Here's how the part is built. I have some questions about the finished solid (model axes, mm). Face numbers are marked on the shaded views. A direction names the side the tool comes from. Round coordinates to 2 decimals unless told otherwise and drop trailing zeros. Order: outer loops, then holes, each group sorted by start corner. A loop starts at its lowest first (then second) coordinate and runs counter-clockwise, first axis right, second up. Notation, with made-up numbers: (43, 80) -> (101, 80) arc R19 cw to (101, 111) -> close; hole circle Ø4 at (42.5, -0.5). An arc over 180 degrees is marked (long way). Use a Markdown table: item, result. Add a question column.
(1) I want a section at A-A, the plane y = 35.5. Please give me the cut outline in (x, z).
(2) I want a section at C-C, the plane x = -35.5. Please give me the cut outline in (y, z), then the cut area to 3 significant figures.
(3) On a 3-axis mill with a long thin cutter (end or side, diameter ignored), from which of +Z, -Z, +X, -X, +Y, -Y can I reach the whole of each face in a straight line? I mean the marked faces 1, 2 and 3. Say none if no direction works.
(4) If I drill on probe 1 along X at (y, z) = (-35.5, -12.5); probe 2 along Y at (x, z) = (48, 25); probe 3 along Z at (x, y) = (-34, -60.5), over which ranges is the centre line in solid material (lowest first)?
(5) I'm going to push flat-ended pins straight in: P1, Ø3.5, axis at x = -38.5, z = 2.5, coming from the +Y side; P2, Ø12, axis at y = 14.5, z = 35.5, coming from the -X side; P3, Ø8, axis at x = 44.5, z = 17.5, coming from the -Y side. Where does each tip first touch, or does it pass through?
(6) I want a section at B-B, the plane z = 64.5. Please give me the cut outline in (x, y).
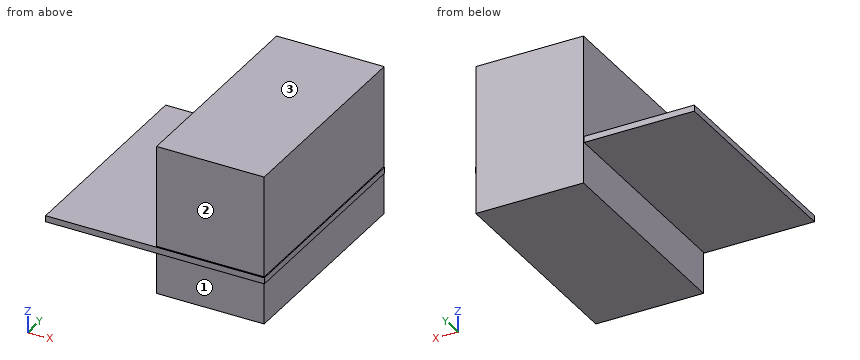
from build123d import *

# Parameters (mm, degrees)
F0_W     = 154.1122123599
F0_H     = 152.2873193026
F1_DEPTH = 4.3168757111
F2_W     = 152.1053090692
F2_H     = 75.8531913161
F3_DEPTH = 25.4
F4_DEPTH = 105.2890252322
F5_DEPTH = 75.802506879


with BuildPart() as f1:
    # F0 (on Top) → F1 (new body)
    with BuildSketch(Plane.XY):
        with Locations((-0.5999542773, -0.8949711919)):
            Rectangle(F0_W, F0_H)
    extrude(amount=F1_DEPTH)

    # F2 (on Right) → F3 (join)
    with BuildSketch(Plane.YZ):
        with Locations((0.0062547624, 37.9265956581)):
            Rectangle(F2_W, F2_H)
    extrude(amount=F3_DEPTH)

    # F4 (add): a face of the model
    f4_faces = [f1.faces().sort_by_distance(p)[0] for p in [
        (12.7, 0.0062547624, 75.8531913161),
    ]]
    extrude(f4_faces, amount=-F4_DEPTH)

    # F5 (add): a face of the model
    f5_faces = [f1.faces().sort_by_distance(p)[0] for p in [
        (0, 0.0234783223, 24.1036447815),
    ]]
    extrude(f5_faces, amount=-F5_DEPTH)


solid = f1.part
Taken from the geometry:
| question | item | result |
|---|---|---|
| 1 | outline | (-77.66, 0) -> (0, 0) -> (0, -29.44) -> (75.8, -29.44) -> (75.8, 0) -> (76.46, 0) -> (76.46, 4.32) -> (75.8, 4.32) -> (75.8, 75.85) -> (0, 75.85) -> (0, 4.32) -> (-77.66, 4.32) -> close |
| 2 | outline | (-77.04, 0) -> (75.25, 0) -> (75.25, 4.32) -> (-77.04, 4.32) -> close |
| 2 | area | 657 mm2 |
| 3 | face 1 | -Z, +X, -X, -Y |
| 3 | face 2 | +Z, +X, -X, -Y |
| 3 | face 3 | +Z, +X, -X, +Y, -Y |
| 4 | probe 1 | x = 0 to 75.8 |
| 4 | probe 2 | y = -76.05 to 76.06 |
| 4 | probe 3 | z = 0 to 4.32 |
| 5 | P1 | stops at y = 75.25 |
| 5 | P2 | stops at x = 0 |
| 5 | P3 | stops at y = -76.05 |
| 6 | outline | (0, -76.05) -> (75.8, -76.05) -> (75.8, 76.06) -> (0, 76.06) -> close |
